Read the model definition and answer for the solid it produces. Units are mm, in the model's axes. A direction names the side the tool comes from. Coordinates: 2 decimals unless noted, no trailing zeros. Write each loop counter-clockwise with the first axis right and the second up, starting at its lowest first coordinate (ties: lowest second). Pieces come first, ordered by that corner, then holes. Notation, with made-up numbers: (51, -5) -> (96, -5) arc R15 ccw to (96, -1) -> close; hole circle Ø3 at (-16.75, -1). An arc over 180 degrees is marked (long way). Answer as a JSON object with one key per item and string values. Group by question number.
(1) Find section C-C (z = 8.75). Give the vertices of the cut face in (x, y) (3 decimals), then the cut area to 3 significant figures.
(2) Straight lines are drawn through the part: L1, parallel to Y at x = -6.25, z = 2.75; L2, parallel to X at y = -14, z = 5.25; L3, parallel to Y at x = -4.25, z = 8.5. For each, find the intervals that lie inside material, in ascending order.
(3) For a pull along X with two mould halves and no side action, classify faces 4 (the face through (-11.373, 21.977, 3.755)), 5 (the face through (-6.382, 15.007, 3.219)), 6 (the face through (0, 0, 5)) as +X half, -X half, draft (parallel to the pull), parting line (faces both ways), or undercut.
(4) Flat-ended cylindrical pins translate along their axes: P1, Ø3, axis at x = -3.5, z = 4.5, coming from the +Y side; P2, Ø3, axis at y = 24.5, z = 2.5, coming from the +X side (3 decimals); P3, Ø1.5, axis at y = 22.75, z = 4.76, coming from the +X side; P4, Ø1.5, axis at y = -6, z = 3.5, coming from the -X side. Find the tip coordinate at first contact, or state that the pin passes through.
(5) Find section B-B (z = 2). Give the vertices of the cut face in (x, y) (3 decimals).
(6) Find section A-A (y = 22.75). Give the vertices of the cut face in (x, z) (1 decimal).
(7) Which of the six approach directions +Z, -Z, +X, -X, +Y, -Y give full straight-line access (tool end or side, diameter ignored) to faces 1 (the face through (-2, -17.75, 5)), 2 (the face through (-6, -11.75, 5)), 3 (the face through (2, 0, 0))?
(8) Find section D-D (x = 2.5). Give the vertices of the cut face in (y, z) (3 decimals).
from build123d import *

# Parameters (mm, degrees)
BOSS_EXTRUDE1_DEPTH             = 9.525
F_2_CLEARANCE_HOLE1_D           = 2.032
F_2_CLEARANCE_HOLE1_DEPTH       = 6.35
F_2_CLEARANCE_HOLE1_TIP         = 0.610474389
F_3_CLEARANCE_HOLE2_D           = 2.54
F_3_CLEARANCE_HOLE2_CSINK_D     = 4.318
F_3_CLEARANCE_HOLE2_CSINK_ANGLE = 90


with BuildPart() as part:
    # Sketch1 → Boss-Extrude1 (new body)
    with BuildSketch(Plane.XY):
        Polygon((0, 11.75), (0, -11.75), (-12.5, -11.75), (-12.5, -27.75), (-9.325, -27.75), (-9.325, -17.75), (5, -17.75), (5, 17.75), (-9.325, 17.75), (-9.325, 27.75), (-12.5, 27.75), (-12.5, 11.75), align=None)
    extrude(amount=BOSS_EXTRUDE1_DEPTH)

    # #2 Clearance Hole1
    with Locations(Plane(origin=(0, 0, 0), x_dir=(-1, 0, 0), z_dir=(0, 0, -1))):
        with Locations((6.25, 14), (6.25, -14)):
            Hole(F_2_CLEARANCE_HOLE1_D / 2, depth=F_2_CLEARANCE_HOLE1_DEPTH)
            with Locations((0, 0, -(F_2_CLEARANCE_HOLE1_DEPTH + F_2_CLEARANCE_HOLE1_TIP / 2))):  # 118° drill point
                Cone(0, F_2_CLEARANCE_HOLE1_D / 2, F_2_CLEARANCE_HOLE1_TIP, mode=Mode.SUBTRACT)

    # #3 Clearance Hole2 (through all)
    with Locations(Plane(origin=(-9.325, 0, 0), x_dir=(0, 0, -1), z_dir=(1, 0, 0))):
        with Locations((-4.7625, 22.75), (-4.7625, -22.75)):
            CounterSinkHole(F_3_CLEARANCE_HOLE2_D / 2, F_3_CLEARANCE_HOLE2_CSINK_D / 2, counter_sink_angle=F_3_CLEARANCE_HOLE2_CSINK_ANGLE)


solid = part.part
Results below:
{
 "1": {"outline": "(-12.5, -27.75) -> (-9.325, -27.75) -> (-9.325, -17.75) -> (5, -17.75) -> (5, 17.75) -> (-9.325, 17.75) -> (-9.325, 27.75) -> (-12.5, 27.75) -> (-12.5, 11.75) -> (0, 11.75) -> (0, -11.75) -> (-12.5, -11.75) -> close", "area": "391 mm2"},
 "2": {"L1": "y = -17.75 to -15.02, -12.98 to -11.75, 11.75 to 12.98, 15.02 to 17.75", "L2": "x = -12.5 to -7.27, -5.23 to 5", "L3": "y = -17.75 to -11.75, 11.75 to 17.75"},
 "3": {"face 4": "draft", "face 5": "undercut", "face 6": "-X half"},
 "4": {"P1": "stops at y = 17.75", "P2": "stops at x = -9.325", "P3": "passes through", "P4": "stops at x = 0"},
 "5": {"outline": "(-12.5, -27.75) -> (-9.325, -27.75) -> (-9.325, -17.75) -> (5, -17.75) -> (5, 17.75) -> (-9.325, 17.75) -> (-9.325, 27.75) -> (-12.5, 27.75) -> (-12.5, 11.75) -> (0, 11.75) -> (0, -11.75) -> (-12.5, -11.75) -> close; hole circle Ø2.032 at (-6.25, -14); hole circle Ø2.032 at (-6.25, 14)"},
 "6": {"outline": "(-12.5, 0) -> (-9.3, 0) -> (-9.3, 2.6) -> (-10.2, 3.5) -> (-12.5, 3.5) -> close; (-12.5, 6) -> (-10.2, 6) -> (-9.3, 6.9) -> (-9.3, 9.5) -> (-12.5, 9.5) -> close"},
 "7": {"face 1": "+Z, -Z, +X, -Y", "face 2": "+Z, -Z, -X", "face 3": "-Z, +X, -X, +Y, -Y"},
 "8": {"outline": "(-17.75, 0) -> (17.75, 0) -> (17.75, 9.525) -> (-17.75, 9.525) -> close"}
}
